from build123d import *

# Parameters (mm, degrees)
SKETCH1_R               = 2.38125
BOSS_EXTRUDE1_DEPTH     = 31.75
CUT_EXTRUDE3_DEPTH      = 32.928094261
CUT_EXTRUDE3_DEPTH_BACK = 32.928094261
SKETCH4_R               = 0.762
CUT_EXTRUDE4_DEPTH      = 32.928094375
CUT_EXTRUDE4_DEPTH_BACK = 32.928094375
SKETCH5_R               = 0.8001


with BuildPart() as part:
    # Sketch1 → Boss-Extrude1 (new, symmetric)
    with BuildSketch(Plane.XY):
        Circle(SKETCH1_R)
    extrude(amount=BOSS_EXTRUDE1_DEPTH, both=True)

    # Sketch4 → Cut-Extrude3 (cut, two sides: drawn at the far end of the back side and taken through both)
    with BuildSketch(Plane(origin=(0, 0, 0), x_dir=(0, 0, -1), z_dir=(1, 0, 0)).offset(-CUT_EXTRUDE3_DEPTH_BACK)):
        with Locations((-22.2885, 0)):
            Circle(SKETCH4_R)
    extrude(amount=CUT_EXTRUDE3_DEPTH + CUT_EXTRUDE3_DEPTH_BACK, mode=Mode.SUBTRACT)

    # Sketch5 → Cut-Extrude4 (cut, two sides: drawn at the far end of the back side and taken through both)
    with BuildSketch(Plane(origin=(0, 0, 0), x_dir=(0, 0, -1), z_dir=(1, 0, 0)).offset(-CUT_EXTRUDE4_DEPTH_BACK)):
        with Locations((23.641617285, 0)):
            Circle(SKETCH5_R)
    extrude(amount=CUT_EXTRUDE4_DEPTH + CUT_EXTRUDE4_DEPTH_BACK, mode=Mode.SUBTRACT)


solid = part.part
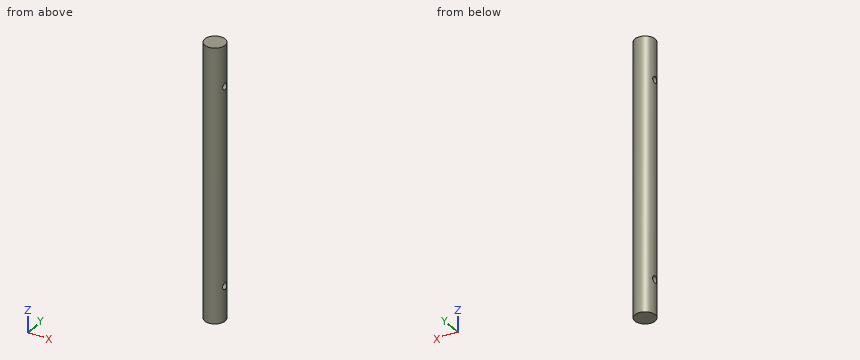
Geometry check sheet. Reference: the model listing, model coordinates, mm. Give positions to 0.01 mm unless a question says otherwise; leave off trailing zeros. Order: outer loops, then holes, each group sorted by start corner. A loop starts at its lowest first (then second) coordinate and runs counter-clockwise, first axis right, second up. Notation, with made-up numbers: (63.25, 18.5) - (75.25, 18.5) arc R14 cw to (75.25, 37.5) - close; hole circle Ø6 at (28, 10.5). An arc over 180 degrees is marked (long way). Answer as a JSON object with one key per item and string values.
(1) Material ranges on line 1 (Z direction, x = -0.9, y = 0); line 2 (Z direction, x = -0.55, y = -0.1); line 3 (Y direction, x = 0.15, z = 25.5), recorded low to high.
Report:
{"line 1": "-31.75 to -24.44, -22.84 to 21.53, 23.05 to 31.75", "line 2": "-31.75 to -24.44, -22.85 to 21.53, 23.04 to 31.75", "line 3": "-2.38 to 2.38"}
(2) Cross-section at C-C (z = -11). Record the cut outline in (x, y), then the cut area to 3 significant figures.
Report:
{"outline": "circle Ø4.76 at (0, 0)", "area": "17.8 mm^2"}
(3) Cross-section at B-B (x = -1.8). Record the cut outline in (y, z), then the cut area to 3 significant figures.
Report:
{"outline": "(-1.56, -31.75) - (1.56, -31.75) - (1.56, 31.75) - (-1.56, 31.75) - close; hole circle Ø1.6 at (0, -23.64); hole circle Ø1.52 at (0, 22.29)", "area": "194 mm^2"}
(4) Depth check by flat-ended pin: pin 1 Ø1.2 at (y, z) = (0, 22.29) entering from +X; pin 2 Ø2.5 at (y, z) = (0, -23.64) entering from -X. Enter the tip coordinate at first touch or a pass-through.
Report:
{"pin 1": "through", "pin 2": "x = -2.38"}
(5) Cross-section at A-A (y = 0). Record the cut outline in (x, z), then the cut area to 3 significant figures.
Report:
{"outline": "(-2.38, -31.75) - (2.38, -31.75) - (2.38, -24.44) - (-2.38, -24.44) - close; (-2.38, -22.84) - (2.38, -22.84) - (2.38, 21.53) - (-2.38, 21.53) - close; (-2.38, 23.05) - (2.38, 23.05) - (2.38, 31.75) - (-2.38, 31.75) - close", "area": "288 mm^2"}
